Source: three-view drawing plus pictorial views. Frame: mm from the lowest corner of the part. A direction names the side the tool comes from. Give positions to 0.01 mm unless a question says otherwise; leave off trailing zeros. Loops run counter-clockwise (first coordinate to the right, second up) from the corner with the lowest first, then second, coordinate; pieces in that order, holes last.
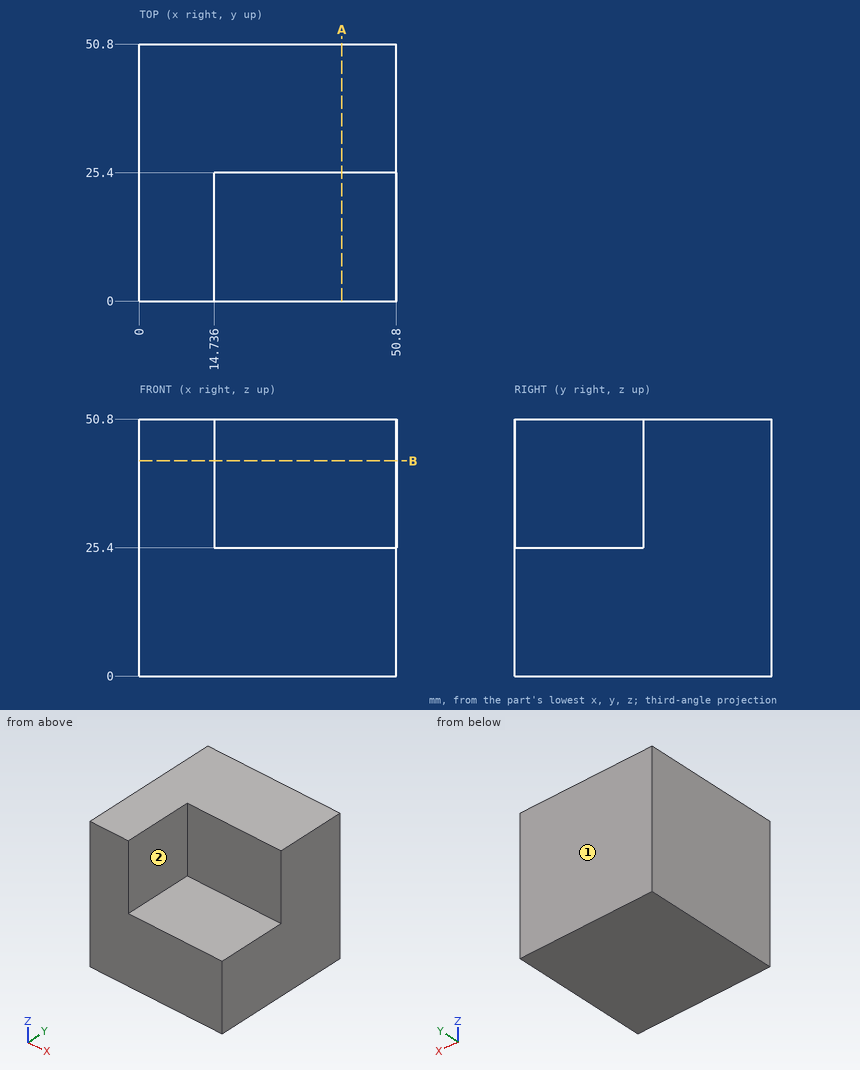
Q1. Section query B-B, the plane z = 42.5. Return loops of the section in (x, y) (1 decimal).
Q2. Pin query (flat end, axial travel): pin 1 Ø6 at (x, z) = (35.5, 44.5) entering from -Y; pin 2 Ø7.5 at (x, y) = (36.5, 7.5) entering from +Z; pin 3 Ø12.5 at (y, z) = (12.5, 36) entering from +X. Return the tip coordinate at first contact, or that it passes through.
Q3. Reachability of the marked faces 1 and 2 from +Z, -Z, +X, -X, +Y, -Y: full face, straight path, thin tool, end or side. Return the list, or none.
Q4. Section query A-A, the plane x = 40. Return loops of the section in (y, z), and give its area (3 significant figures).
Q5. Material intervals for probe 1 along Y at (x, z) = (31.5, 32.5); probe 2 along Z at (x, y) = (38.5, 13); probe 3 along X at (y, z) = (13, 45) (1 decimal), sorted ascending.
Resolved:
1. outline: (0, 0) - (14.7, 0) - (14.7, 25.4) - (50.8, 25.4) - (50.8, 50.8) - (0, 50.8) - close
2. pin 1: stops at y = 25.4
2. pin 2: stops at z = 25.4
2. pin 3: stops at x = 14.74
3. face 1: +Z, -Z, +X, -X, +Y
3. face 2: +Z, +X, -Y
4. outline: (0, 0) - (50.8, 0) - (50.8, 50.8) - (25.4, 50.8) - (25.4, 25.4) - (0, 25.4) - close
4. area: 1,940 mm2
5. probe 1: y = 25.4 to 50.8
5. probe 2: z = 0 to 25.4
5. probe 3: x = 0 to 14.7
